Geometry: final body of the model. Coordinates: model frame, mm. A direction names the side the tool comes from. Coordinates: 2 decimals unless noted, no trailing zeros. Order: outer loops, then holes, each group sorted by start corner. A loop starts at its lowest first (then second) coordinate and runs counter-clockwise, first axis right, second up. Notation, with made-up numbers: (-4, 87.5) -> (7, 87.5) arc R9 ccw to (7, 91.5) -> close; hole circle Ø9 at (-39, -12). An arc over 180 degrees is marked (long way). Answer in a Markdown table with one row per item. Add a question column.
1) Ray query, line 1 (X direction, y = 3.75, z = 2.85); line 2 (Y direction, x = 39, z = 1.85); line 3 (X direction, y = 19.5, z = 2.55). Return the intervals inside material, ascending. Write a range as from..to.
2) Contact query for a flat-ended pin moving along its axis: P1, Ø1.8, axis at y = 3, z = 3, coming from the -X side. Output: stop coordinate, or through.
3) Section query A-A on z = 4. Return the cut outline in (x, y).
4) Pull-direction query (X, two-part tool) for faces 1 (the face through (6, 20, 3)), 2 (the face through (52.5, 3, 3)), 3 (the face through (47, 12, 6)), 4 (the face through (26, 6, 3)); classes: +X half, -X half, draft (parallel to the pull), parting line (faces both ways), or undercut.
5) Section query B-B on y = 17. Return the cut outline in (x, z).
6) Set-up query: faces 5 (the face through (8.89, 18.01, 3.04)), 6 (the face through (3, 18, 3)), 7 (the face through (92, 18, 3)), 8 (the face through (85, 3, 3)), 9 (the face through (90, 0, 3)). Return all of +Z, -Z, +X, -X, +Y, -Y with unobstructed straight access to the full face (end or side cutting, diameter ignored); none if empty.
7) Section query C-C on x = 69. Return the cut outline in (y, z).
```python
from build123d import *

# Parameters (mm, degrees)
SKETCH1_W           = 95
SKETCH1_H           = 23
BOSS_EXTRUDE1_DEPTH = 6
SKETCH2_W           = 32.5
SKETCH2_H           = 6
CUT_EXTRUDE1_DEPTH  = 7
SKETCH4_R           = 1.5
CUT_EXTRUDE2_DEPTH  = 7
SKETCH5_W           = 6
SKETCH5_H           = 5
CUT_EXTRUDE3_DEPTH  = 7


with BuildPart() as part:
    # Sketch1 → Boss-Extrude1 (new body)
    with BuildSketch(Plane.XY):
        with Locations((47.5, 11.5)):
            Rectangle(SKETCH1_W, SKETCH1_H)
    extrude(amount=BOSS_EXTRUDE1_DEPTH)

    # Sketch2 → Cut-Extrude1 (cut, through all)
    with BuildSketch(Plane.XY.offset(6)):
        with Locations((26.25, 3)):
            Rectangle(SKETCH2_W, SKETCH2_H)
        with Locations((68.75, 3)):
            Rectangle(SKETCH2_W, SKETCH2_H)
    extrude(amount=-CUT_EXTRUDE1_DEPTH, mode=Mode.SUBTRACT)

    # Sketch4 → Cut-Extrude2 (cut, through all)
    with BuildSketch(Plane.XY.offset(6)):
        with Locations((10, 17)):
            Circle(SKETCH4_R)
        with Locations((85, 17)):
            Circle(SKETCH4_R)
    extrude(amount=-CUT_EXTRUDE2_DEPTH, mode=Mode.SUBTRACT)

    # Sketch5 → Cut-Extrude3 (cut, through all)
    with BuildSketch(Plane.XY.offset(6)):
        with Locations((3, 20.5)):
            Rectangle(SKETCH5_W, SKETCH5_H)
        with Locations((92, 20.5)):
            Rectangle(SKETCH5_W, SKETCH5_H)
    extrude(amount=-CUT_EXTRUDE3_DEPTH, mode=Mode.SUBTRACT)


solid = part.part
```
Result:
| question | item | result |
|---|---|---|
| 1 | line 1 | 0..10, 42.5..52.5, 85..95 |
| 1 | line 2 | 6..23 |
| 1 | line 3 | 6..89 |
| 2 | P1 | x = 0 |
| 3 | outline | (0, 0) -> (10, 0) -> (10, 6) -> (42.5, 6) -> (42.5, 0) -> (52.5, 0) -> (52.5, 6) -> (85, 6) -> (85, 0) -> (95, 0) -> (95, 18) -> (89, 18) -> (89, 23) -> (6, 23) -> (6, 18) -> (0, 18) -> close; hole circle Ø3 at (10, 17); hole circle Ø3 at (85, 17) |
| 4 | face 1 | -X half |
| 4 | face 2 | undercut |
| 4 | face 3 | draft |
| 4 | face 4 | undercut |
| 5 | outline | (0, 0) -> (8.5, 0) -> (8.5, 6) -> (0, 6) -> close; (11.5, 0) -> (83.5, 0) -> (83.5, 6) -> (11.5, 6) -> close; (86.5, 0) -> (95, 0) -> (95, 6) -> (86.5, 6) -> close |
| 6 | face 5 | +Z, -Z |
| 6 | face 6 | +Z, -Z, -X, +Y |
| 6 | face 7 | +Z, -Z, +X, +Y |
| 6 | face 8 | +Z, -Z, -Y |
| 6 | face 9 | +Z, -Z, +X, -X, -Y |
| 7 | outline | (6, 0) -> (23, 0) -> (23, 6) -> (6, 6) -> close |
